Input: part model. Units: mm. Frame: model coordinates. Face numbers are marked on the shaded views. A direction names the side the tool comes from. Coordinates: 2 decimals unless noted, no trailing zeros. Order: outer loops, then holes, each group sorted by start corner. A loop starts at its lowest first (then second) coordinate and runs counter-clockwise, first axis right, second up. Notation, with made-up numbers: (87, -23) -> (141, -23) arc R32 ccw to (141, 8) -> close; hole circle Ø8 at (73, 54.5). An arc over 180 degrees is marked (long way). Use one line per item in the form item = value. Start each with the question number.
1) Ray query, line 1 along Z through (x, y) = (6, 4.5); line 2 along Z through (x, y) = (2.25, 9); line 3 along Y through (x, z) = (1.5, 10). Return the intervals inside material, ascending.
2) Section query B-B on z = 23.5. Output: boundary loops of the cut face in (x, y), then the cut area to 3 significant figures.
3) Section query D-D on y = -2. Output: boundary loops of the cut face in (x, z), then the cut area to 3 significant figures.
4) Section query A-A on y = 4.75. Output: boundary loops of the cut face in (x, z).
5) Draft query along Z for the marked faces 1, 2 and 3. Return one class per face: pulls with the +Z half, pulls with the -Z half, needs draft (parallel to the pull), parting line crosses it, or undercut.
6) Pin query (flat end, axial travel): pin 1 (10 mm diameter, centred on x = 15, z = 14.5, fed in from -Y); pin 2 (11 mm diameter, centred on x = 16, z = 15, fed in from +Y); pin 3 (1 mm diameter, centred on x = 14.5, y = -2, fed in from +Z); pin 4 (5 mm diameter, centred on x = 15, z = 19.5, fed in from +Y). Return the tip coordinate at first contact, or that it passes through.
7) Access query for the marked faces 4, 5 and 6. Directions: +Z, -Z, +X, -X, +Y, -Y. A direction counts if a zero-diameter tool reaches every point of the face in a straight line with its end or side. Return the directions, or none.
8) Section query C-C on x = 8.25. Output: boundary loops of the cut face in (y, z).
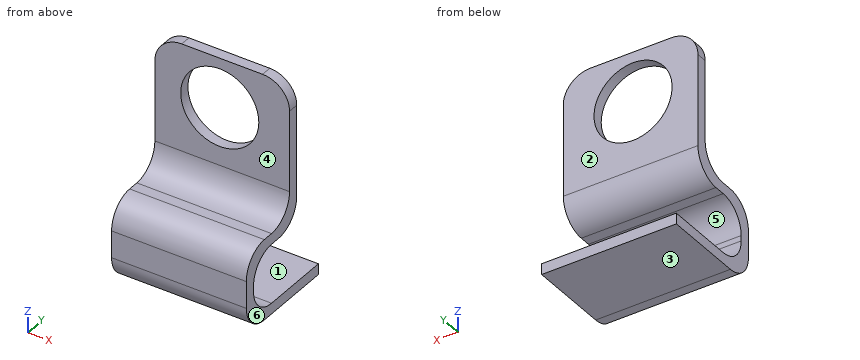
from build123d import *

# Parameters (mm, degrees)
F1_DEPTH = 25
F2_R     = 5
F3_R     = 7.25
F4_DEPTH = 25


with BuildPart() as f1:
    # F0 (on Right) → F1 (new body)
    with BuildSketch(Plane.YZ):
        Polygon((6.056661, 29.318909), (4.056661, 29.318909), (4.056661, 4.318909), (-7.943339, 4.318909), (-7.943339, -10.681091), (12.056661, -10.681091), (12.06602, -8.681091), (-5.943339, -8.681091), (-5.943339, 2.318909), (6.056661, 2.318909), align=None)
    extrude(amount=F1_DEPTH)

    # F2
    f2_edges = [f1.edges().sort_by_distance(p)[0] for p in [
        (12.5, 4.056661, 4.318909),
        (12.5, -7.943339, 4.318909),
        (12.5, -7.943339, -10.681091),
        (12.5, -5.943339, 2.318909),
        (12.5, -5.943339, -8.681091),
        (12.5, 6.056661, 2.318909),
        (25, 5.056661, 29.318909),
        (0, 5.056661, 29.318909),
    ]]
    fillet(f2_edges, radius=F2_R)

    # F3 (on Front) → F4 (cut)
    with BuildSketch(Plane.XZ):
        with Locations((12.048211, 20.089075)):
            Circle(F3_R)
    extrude(amount=-F4_DEPTH, mode=Mode.SUBTRACT)


solid = f1.part
Answers below:
q1.line_1 = -10.68 to -8.68, 3.69 to 16.09, 24.09 to 29.32
q1.line_2 = -10.68 to -8.68
q1.line_3 = 4.06 to 6.06
q2.outline = (0, 4.06) -> (5.65, 4.06) -> (5.65, 6.06) -> (0, 6.06) -> close; (18.45, 4.06) -> (25, 4.06) -> (25, 6.06) -> (18.45, 6.06) -> close
q2.area = 24.4 mm^2
q3.outline = (0, -10.68) -> (25, -10.68) -> (25, -8.57) -> (0, -8.57) -> close; (0, 2.21) -> (25, 2.21) -> (25, 4.32) -> (0, 4.32) -> close
q3.area = 106 mm^2
q4.outline = (0, -10.68) -> (25, -10.68) -> (25, -8.68) -> (0, -8.68) -> close; (0, 3.95) -> (25, 3.95) -> (25, 24.32) arc R5 ccw to (20, 29.32) -> (5, 29.32) arc R5 ccw to (0, 24.32) -> close; hole circle Ø14.5 at (12.05, 20.09)
q5.face_1 = undercut
q5.face_2 = needs draft
q5.face_3 = pulls with the -Z half
q6.pin_1 = 4.06
q6.pin_2 = 6.06
q6.pin_3 = 4.32
q6.pin_4 = through
q7.face_4 = +Z, +X, -X, -Y
q7.face_5 = +X, -X, +Y
q7.face_6 = +Z, -Z, +X, +Y, -Y
q8.outline = (-7.94, -5.68) arc R5 ccw to (-2.94, -10.68) -> (12.06, -10.68) -> (12.07, -8.68) -> (-0.94, -8.68) arc R5 cw to (-5.94, -3.68) -> (-5.94, -2.68) arc R5 cw to (-0.94, 2.32) -> (1.06, 2.32) arc R5 ccw to (6.06, 7.32) -> (6.06, 13.91) -> (4.06, 13.91) -> (4.06, 9.32) arc R5 cw to (-0.94, 4.32) -> (-2.94, 4.32) arc R5 ccw to (-7.94, -0.68) -> close; (4.06, 26.26) -> (6.06, 26.26) -> (6.06, 29.32) -> (4.06, 29.32) -> close
